```python
from build123d import *

# Parameters (mm, degrees)
BOSS_EXTRUDE1_DEPTH = 60
FILLET1_R           = 0.5
SKETCH3_R           = 1.000778627
CUT_EXTRUDE1_DEPTH  = 60
SKETCH4_R           = 1.000778627
BOSS_EXTRUDE2_DEPTH = 50
FILLET2_R           = 0.5


with BuildPart() as part:
    # Sketch2 → Boss-Extrude1 (new body)
    with BuildSketch(Plane(origin=(0, 0, 0), x_dir=(1, 0, 0), z_dir=(0, 1, 0))):
        with BuildLine():
            Line((22, -1.5), (22, 1.5))
            Line((22, 1.5), (2, 1.5))
            ThreePointArc((2, 1.5), (1.767766953, 1.767766953), (1.5, 2))
            Line((1.5, 2), (1.5, 22))
            Line((1.5, 22), (-1.5, 22))
            Line((-1.5, 22), (-1.5, 2))
            ThreePointArc((-1.5, 2), (-1.767766953, 1.767766953), (-2, 1.5))
            Line((-2, 1.5), (-22, 1.5))
            Line((-22, 1.5), (-22, -1.5))
            Line((-22, -1.5), (-2, -1.5))
            ThreePointArc((-2, -1.5), (-1.767766953, -1.767766953), (-1.5, -2))
            Line((-1.5, -2), (-1.5, -22))
            Line((-1.5, -22), (1.5, -22))
            Line((1.5, -22), (1.5, -2))
            ThreePointArc((1.5, -2), (1.767766953, -1.767766953), (2, -1.5))
            Line((2, -1.5), (22, -1.5))
        make_face()
    extrude(amount=BOSS_EXTRUDE1_DEPTH)

    # Fillet1
    fillet1_edges = [part.edges().sort_by_distance(p)[0] for p in [
        (22, 0, 0),
        (0, 0, 22),
        (0, 60, -22),
        (-22, 0, 0),
        (0, 0, -22),
        (22, 30, -1.5),
        (22, 30, 1.5),
        (1.5, 30, 22),
        (-1.5, 30, 22),
        (-22, 30, 1.5),
        (-22, 30, -1.5),
        (-1.5, 30, -22),
        (1.5, 30, -22),
        (-22, 60, 0),
        (0, 60, 22),
        (22, 60, 0),
    ]]
    fillet(fillet1_edges, radius=FILLET1_R)

    # Sketch3 → Cut-Extrude1 (cut)
    with BuildSketch(Plane(origin=(0, 0, 0), x_dir=(1, 0, 0), z_dir=(0, 1, 0))):
        with Locations(Location((0, 0, 0), (0, 0, 270))):
            Circle(SKETCH3_R)
    extrude(amount=CUT_EXTRUDE1_DEPTH, mode=Mode.SUBTRACT)

    # Sketch4 → Boss-Extrude2 (add, symmetric)
    with BuildSketch(Plane(origin=(0, 30, 0), x_dir=(1, 0, 0), z_dir=(0, 1, 0))):
        with Locations(Location((0, 0, 0), (0, 0, 270))):
            Circle(SKETCH4_R)
    extrude(amount=BOSS_EXTRUDE2_DEPTH, both=True)

    # Fillet2
    fillet2_edges = [part.edges().sort_by_distance(p)[0] for p in [
        (0, 60, -1.000778627),
        (0, 0, -1.000778627),
    ]]
    fillet(fillet2_edges, radius=FILLET2_R)


solid = part.part
```
Geometry check sheet. Reference: the model listing, model coordinates, mm. A direction names the side the tool comes from. Coordinates: 2 decimals unless noted, no trailing zeros. Order: outer loops, then holes, each group sorted by start corner. A loop starts at its lowest first (then second) coordinate and runs counter-clockwise, first axis right, second up.
Item 1: Scan lines: line 1 along Z through (x, y) = (20, 15); line 2 along Y through (x, z) = (8, 0). Record each from-to range of solid material in increasing order.
Item 2: Section check D-D (z = -19). Enter the section's corners in (x, y).
Item 3: Depth check by flat-ended pin: pin 1 (1 mm diameter, centred on x = 12, y = 13.5, fed in from -Z); pin 2 (21.5 mm diameter, centred on x = -10.5, z = -10.5, fed in from -Y); pin 3 (12 mm diameter, centred on y = 7, z = -12.5, fed in from -X); pin 4 (4 mm diameter, centred on x = -7, z = -5, fed in from +Y). Enter the tip coordinate at first touch or a pass-through.
Item 4: Section check B-B (x = 0). Enter the section's corners in (y, z).
Item 5: Section check A-A (z = 0). Enter the section's corners in (x, y), plus the area to 3 significant figures.
Item 6: Tool access check on faces 1 (the flat face through (1.5, 30, -12)), 2 (the flat face through (-1.5, 30, 12)), 3 (the flat face through (1.5, 30, 12)), 4 (the flat face through (-1.5, 30, -12)). Record the directions out of +Z, -Z, +X, -X, +Y, -Y that give a thin tool (end or side, any length) a straight path to the whole face; none if there is none.
Item 7: Section check C-C (y = -14). Enter the section's corners in (x, z).
Check sheet entries:
1. line 1: z = -1.5 to 1.5
1. line 2: y = 0 to 60
2. outline: (-1.5, 0) - (1.5, 0) - (1.5, 60) - (-1.5, 60) - close
3. pin 1: stops at z = -1.5
3. pin 2: stops at y = 0
3. pin 3: stops at x = -1.5
3. pin 4: passes through
4. outline: (-20, -1) - (-0.5, -1) arc R0.5 cw to (0, -1.5) - (0, -21.5) arc R0.5 ccw to (0.5, -22) - (59.5, -22) arc R0.5 ccw to (60, -21.5) - (60, -1.5) arc R0.5 cw to (60.5, -1) - (80, -1) - (80, 1) - (60.5, 1) arc R0.5 cw to (60, 1.5) - (60, 21.5) arc R0.5 ccw to (59.5, 22) - (0.5, 22) arc R0.5 ccw to (0, 21.5) - (0, 1.5) arc R0.5 cw to (-0.5, 1) - (-20, 1) - close
5. outline: (-22, 0.5) arc R0.5 ccw to (-21.5, 0) - (-1.5, 0) arc R0.5 cw to (-1, -0.5) - (-1, -20) - (1, -20) - (1, -0.5) arc R0.5 cw to (1.5, 0) - (21.5, 0) arc R0.5 ccw to (22, 0.5) - (22, 59.5) arc R0.5 ccw to (21.5, 60) - (1.5, 60) arc R0.5 cw to (1, 60.5) - (1, 80) - (-1, 80) - (-1, 60.5) arc R0.5 cw to (-1.5, 60) - (-21.5, 60) arc R0.5 ccw to (-22, 59.5) - close
5. area: 2,720 mm2
6. face 1: -Z, +X, +Y, -Y
6. face 2: +Z, -X, +Y, -Y
6. face 3: +Z, +X, +Y, -Y
6. face 4: -Z, -X, +Y, -Y
7. outline: circle Ø2 at (0, 0)
